Geometry: final body of the model. Coordinates: model frame, mm. A direction names the side the tool comes from. Give positions to 0.01 mm unless a question says otherwise; leave off trailing zeros. Write each loop counter-clockwise with the first axis right and the second up, starting at its lowest first coordinate (ties: lowest second). Pieces come first, ordered by that corner, then holes. Notation, with made-up numbers: (30.5, 27) - (76.5, 27) arc R8 ccw to (76.5, 38) - close; hole circle Ø1 at (59.5, 75.25). An arc over 180 degrees is marked (long way). Use CSV: the item, a comma, the result in double quotes. Start each with the question number.
(1) Section C-C on y = -0.5. Output: boundary loops of the cut face in (x, z), and give its area (3 significant figures).
(2) Line query: probe 1 along X at (y, z) = (5.5, 7.75); probe 2 along Y at (x, z) = (12.75, 8.75); probe 3 along X at (y, z) = (-5.25, 5). Output: solid intervals per line, ascending. Write a range as [from, to].
(3) First-contact query: pin 1 Ø1.8 at (y, z) = (8.5, 4) entering from +X; pin 2 Ø5 at (y, z) = (-3.5, 5.5) entering from -X. Flat tips, straight axial feed; report the tip coordinate or a pass-through.
(4) Section A-A on z = 4. Output: boundary loops of the cut face in (x, y).
(5) Section B-B on x = 10.5. Output: boundary loops of the cut face in (y, z).
(6) Reachability of faces 1 (the flat face through (4, -3, 5)), 2 (the flat face through (10, 7, 5)), 3 (the flat face through (7, 2, 0)) from +Z, -Z, +X, -X, +Y, -Y: full face, straight path, thin tool, end or side. Return the list, or none.
from build123d import *

# Parameters (mm, degrees)
BOX001_W     = 10
BOX001_H     = 10
BOX001_DEPTH = 10
BOX_W        = 10
BOX_H        = 10
BOX_DEPTH    = 10


with BuildPart() as cubo001:
    # Box001 → Box001 (new body)
    with BuildSketch(Plane(origin=(4, -6, 0), x_dir=(1, 0, 0), z_dir=(0, 0, 1))):
        with Locations((5, 5)):
            Rectangle(BOX001_W, BOX001_H)
    extrude(amount=BOX001_DEPTH)


with BuildPart() as fusion:
    # Box → Box (new body)
    with BuildSketch(Plane.XY):
        with Locations((5, 5)):
            Rectangle(BOX_W, BOX_H)
    extrude(amount=BOX_DEPTH)

    # Fusion: union Cubo001
    add(cubo001.part)


solid = fusion.part
Check values:
1,outline,"(4, 0) - (14, 0) - (14, 10) - (4, 10) - close"
1,area,"100 mm²"
2,probe 1,"x = [0, 10]"
2,probe 2,"y = [-6, 4]"
2,probe 3,"x = [4, 14]"
3,pin 1,"stops at x = 10"
3,pin 2,"stops at x = 4"
4,outline,"(0, 0) - (4, 0) - (4, -6) - (14, -6) - (14, 4) - (10, 4) - (10, 10) - (0, 10) - close"
5,outline,"(-6, 0) - (4, 0) - (4, 10) - (-6, 10) - close"
6,face 1,"+Z, -Z, -X, -Y"
6,face 2,"+Z, -Z, +X, +Y"
6,face 3,"-Z, +X, -X, +Y, -Y"
